Input: part model. Units: mm. Frame: model coordinates. Face numbers are marked on the shaded views. A direction names the side the tool comes from. Coordinates: 2 decimals unless noted, no trailing zeros. Write each loop counter-clockwise with the first axis right and the second up, starting at its lowest first coordinate (ties: lowest second). Pieces come first, ordered by that corner, then holes. Notation, with made-up numbers: M 11.25,85 L 62.25,85 A17 ccw 62.25,91 Z; hole C 0,-16.75 d8. An arc over 180 degrees is marked long. Use one line per item in the form item = value.
from build123d import *

# Parameters (mm, degrees)
BOSS_EXTRUDE1_DEPTH = 100
CUT_EXTRUDE1_REACH  = 42
SKETCH2_W           = 35
SKETCH2_H           = 40
SKETCH3_W           = 20
SKETCH3_H           = 15
BOSS_EXTRUDE2_DEPTH = 45
SKETCH4_W           = 20
SKETCH4_H           = 15
BOSS_EXTRUDE3_DEPTH = 40
BOSS_EXTRUDE4_DEPTH = 15


with BuildPart() as part:
    # Sketch1 → Boss-Extrude1 (new body)
    with BuildSketch(Plane.XY):
        with BuildLine():
            Line((-20, -45.82575695), (-20, -21.010205144))
            Line((-20, -21.010205144), (20, -21.010205144))
            Line((20, -21.010205144), (20, -6.010205144))
            Line((20, -6.010205144), (0, -6.010205144))
            ThreePointArc((0, -6.010205144), (-7.071067812, -3.081272956), (-10, 3.989794856))
            Line((-10, 3.989794856), (-10, 48.989794856))
            ThreePointArc((-10, 48.989794856), (-49.724211568, 5.244309675), (-20, -45.82575695))
        make_face()
    extrude(amount=BOSS_EXTRUDE1_DEPTH)

    # Sketch2 → Cut-Extrude1 (cut, up to next)
    with BuildSketch(Plane(origin=(-10, 0, 0), x_dir=(0, 0, -1), z_dir=(1, 0, 0)), mode=Mode.PRIVATE) as cut_extrude1_sk1:
        with Locations((-52.5, 28.989794856)):
            Rectangle(SKETCH2_W, SKETCH2_H)
    cut_extrude1_tool1 = extrude(cut_extrude1_sk1.sketch, amount=-CUT_EXTRUDE1_REACH, mode=Mode.PRIVATE) & part.part
    add(cut_extrude1_tool1.solids().sort_by_distance((-10, 28.989795, 52.5))[0], mode=Mode.SUBTRACT)

    # Sketch3 → Boss-Extrude2 (add)
    with BuildSketch(Plane.XY.offset(35)):
        with Locations((-15, 26.489794856)):
            Rectangle(SKETCH3_W, SKETCH3_H)
    extrude(amount=-BOSS_EXTRUDE2_DEPTH)

    # Sketch4 → Boss-Extrude3 (add)
    with BuildSketch(Plane(origin=(0, 0, 70), x_dir=(-1, 0, 0), z_dir=(0, 0, -1))):
        with Locations((15, 26.489794856)):
            Rectangle(SKETCH4_W, SKETCH4_H)
    extrude(amount=-BOSS_EXTRUDE3_DEPTH)

    # Sketch5 → Boss-Extrude4 (add)
    with BuildSketch(Plane.XY.offset(100)):
        with BuildLine():
            Line((20, -16.010205144), (-49.987139252, -1.133979464))
            ThreePointArc((-49.987139252, -1.133979464), (-41.519738184, -27.85877494), (-20, -45.82575695))
            Line((-20, -45.82575695), (-20, -21.010205144))
            Line((-20, -21.010205144), (20, -21.010205144))
            Line((20, -21.010205144), (20, -16.010205144))
        make_face()
    extrude(amount=BOSS_EXTRUDE4_DEPTH)


solid = part.part
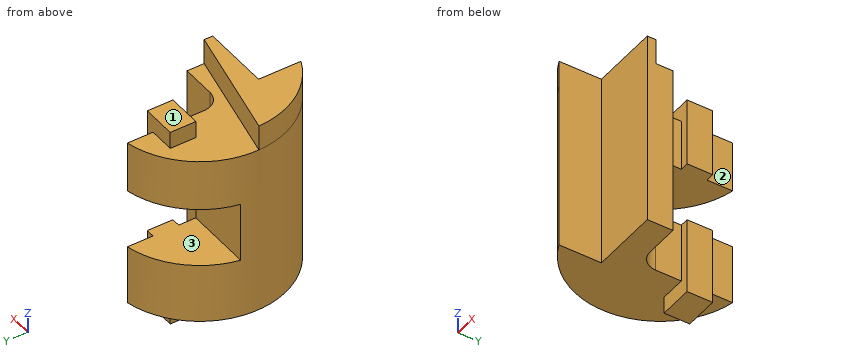
(1) Set-up query: the marked faces 1, 2 and 3. Return all of +Z, -Z, +X, -X, +Y, -Y with unobstructed straight access to the full face (end or side cutting, diameter ignored); none if empty.
Computed:
face_1 = +Z, +X, -X, +Y
face_2 = +Z, -Z, +X, +Y
face_3 = +X, -X, +Y
(2) Section query D-D on x = 9.5. Return the cut outline in (y, z), plus the area to 3 significant figures.
Computed:
outline = M -21.01,0 L -6.01,0 L -6.01,100 L -13.78,100 L -13.78,115 L -21.01,115 Z
area = 1,610 mm^2
(3) Section query A-A on z = 104.5. Return the cut outline in (x, y).
Computed:
outline = M -49.99,-1.13 A50 ccw -20,-45.83 L -20,-21.01 L 20,-21.01 L 20,-16.01 Z; M -25,18.99 L -5,18.99 L -5,33.99 L -25,33.99 Z
(4) Section query B-B on y = 26. Return the cut outline in (x, z), plus the area to 3 significant figures.
Computed:
outline = M -42.71,0 L -25,0 L -25,-10 L -5,-10 L -5,35 L -42.71,35 Z; M -42.71,70 L -5,70 L -5,110 L -25,110 L -25,100 L -42.71,100 Z
area = 2,850 mm^2
(5) First-contact query: pin 1 Ø4.5 at (y, z) = (23, 20.5) entering from +X; pin 2 Ø6 at (x, z) = (9.5, 70) entering from +Y; pin 3 Ø7.5 at (y, z) = (9, 69.5) entering from +X; pin 4 Ø12 at (x, y) = (-10, -31.5) entering from -Z. Flat tips, straight axial feed; report the tip coordinate or a pass-through.
Computed:
pin_1 = -5
pin_2 = -6.01
pin_3 = -10
pin_4 = through
(6) Line query: probe 1 along Z at (x, y) = (-15, 11.5); probe 2 along Z at (x, y) = (3, -8); probe 3 along Z at (x, y) = (-30.5, -16.5). Output: solid intervals per line, ascending.
Computed:
probe_1 = 0 to 35, 70 to 100
probe_2 = 0 to 100
probe_3 = 0 to 115
(7) Section query C-C on z = 8.5. Return the cut outline in (x, y).
Computed:
outline = M -20,-45.83 L -20,-21.01 L 20,-21.01 L 20,-6.01 L 0,-6.01 A10 cw -10,3.99 L -10,18.99 L -5,18.99 L -5,33.99 L -10,33.99 L -10,48.99 A50 ccw Z
